Source: CAD feature listing. Evaluate the final solid. Frame: model axes, mm. A direction names the side the tool comes from. Give positions to 0.01 mm unless a question says otherwise; leave off trailing zeros. Loops run counter-clockwise (first coordinate to the right, second up) from the corner with the lowest first, then second, coordinate; pieces in that order, holes last. Notation, with made-up numbers: M 45.5,87.25 L 57.5,87.25 A34 ccw 57.5,122.25 Z; hole C -37,-36 d3. An arc over 180 degrees is marked long. Put each result on its own line as item: value.
from build123d import *

# Parameters (mm, degrees)
F0_R     = 12.5
F1_DEPTH = 20
F2_DEPTH = 5
F3_R     = 7.5
F4_DEPTH = 50


with BuildPart() as f1:
    # F0 (on Front) → F1 (new body, symmetric)
    with BuildSketch(Plane.XZ):
        with BuildLine():
            Line((63.232286, 3.888947), (37.476556, 3.888947))
            ThreePointArc((37.476556, 3.888947), (29.260214, 26.727902), (11.256595, 43.006594))
            ThreePointArc((11.256595, 43.006594), (-55.988459, 23.157086), (-37.272816, -44.412323))
            Line((-37.272816, -44.412323), (-37.272816, -76.111053))
            Line((-37.272816, -76.111053), (-15.272816, -76.111053))
            Line((-15.272816, -76.111053), (-15.272816, -32.970117))
            ThreePointArc((-15.272816, -32.970117), (-12.272816, 30.888947), (-9.272816, -32.970117))
            Line((-9.272816, -32.970117), (-9.272816, -33.111053))
            Line((-9.272816, -33.111053), (-9.272816, -76.111053))
            Line((-9.272816, -76.111053), (12.727184, -76.111053))
            Line((12.727184, -76.111053), (12.727184, -44.412323))
            ThreePointArc((12.727184, -44.412323), (29.722588, -28.247486), (37.476556, -6.111053))
            Line((37.476556, -6.111053), (63.232286, -6.111053))
            ThreePointArc((63.232286, -6.111053), (107.0921, -16.922441), (87.727184, 23.888947))
            ThreePointArc((87.727184, 23.888947), (71.915795, 18.253864), (63.232286, 3.888947))
        make_face()
        with Locations((87.727184, -1.111053)):
            Circle(F0_R, mode=Mode.SUBTRACT)
    extrude(amount=F1_DEPTH, both=True)

    # F0 (on Front) → F2 (join, symmetric)
    with BuildSketch(Plane.XZ):
        with BuildLine():
            ThreePointArc((11.256595, 43.006594), (29.260214, 26.727902), (37.476556, 3.888947))
            Line((37.476556, 3.888947), (63.232286, 3.888947))
            ThreePointArc((63.232286, 3.888947), (71.915795, 18.253864), (87.727184, 23.888947))
            Line((87.727184, 23.888947), (11.256595, 43.006594))
        make_face()
    extrude(amount=F2_DEPTH, both=True)

    # F3 (on Right) → F4 (cut, symmetric)
    with BuildSketch(Plane.YZ):
        with Locations((0, -58.611053)):
            Circle(F3_R)
    extrude(amount=F4_DEPTH, both=True, mode=Mode.SUBTRACT)


solid = f1.part
1. Section query C-C (x = 80). Output: boundary loops of the cut face in (y, z), plus the area to 3 significant figures.
Found:
outline: M -20,-24.89 L 20,-24.89 L 20,-10.94 L -20,-10.94 Z; M -20,8.71 L 20,8.71 L 20,22.66 L 5,22.66 L 5,25.82 L -5,25.82 L -5,22.66 L -20,22.66 Z
area: 1,150 mm^2
2. Access query for faces 5 (the flat face through (-15.273, 0, -50)), 6 (the flat face through (-37.273, 0, -67)), 7 (the flat face through (49, 5, 24)), 8 (the flat face through (12.727, 0, -68)), 9 (the flat face through (49, -5, 24)). Directions: +Z, -Z, +X, -X, +Y, -Y. A direction counts if a zero-diameter tool reaches every point of the face in a straight line with its end or side. Return the directions, or none.
Found:
face 5: -Z, +Y, -Y
face 6: -Z, -X, +Y, -Y
face 7: +Z, +Y
face 8: -Z, +X, +Y, -Y
face 9: +Z, -Y
3. Draft query along Y for faces 1 (the flat face through (51, 12, 3.889)), 2 (the cylindrical face through (1.881, 3.461, -65.265)), 3 (the flat face through (12, -20, -23)), 4 (the flat face through (12, 20, -23)). Return one class per face: pulls with the +Y half, pulls with the -Y half, needs draft (parallel to the pull), parting line crosses it, or undercut.
Found:
face 1: needs draft
face 2: undercut
face 3: pulls with the -Y half
face 4: pulls with the +Y half
4. Material intervals for line 1 (X direction, y = 12.5, z = 0.5); line 2 (X direction, y = -8, z = -66); line 3 (Z direction, x = 4, y = 0), sorted ascending. Write a range as from..to.
Found:
line 1: -62.25..-44.23, 19.69..75.33, 100.12..112.68
line 2: -37.27..-15.27, -9.27..12.73
line 3: -76.11..-66.11, -51.11..-28.66, 26.44..46.17
5. Section query D-D (z = -36.5). Output: boundary loops of the cut face in (x, y).
Found:
outline: M -47.59,-20 L -15.27,-20 L -15.27,20 L -47.59,20 Z; M -9.27,-20 L 23.05,-20 L 23.05,20 L -9.27,20 Z
6. Section query B-B (y = 0). Output: boundary loops of the cut face in (x, z), plus the area to 3 significant figures.
Found:
outline: M -37.27,-76.11 L -15.27,-76.11 L -15.27,-66.11 L -37.27,-66.11 Z; M -37.27,-51.11 L -15.27,-51.11 L -15.27,-32.97 A32 cw long -9.27,-32.97 L -9.27,-51.11 L 12.73,-51.11 L 12.73,-44.41 A50 ccw 37.48,-6.11 L 63.23,-6.11 A25 ccw long 87.73,23.89 L 11.26,43.01 A50 ccw -37.27,-44.41 Z; M -9.27,-76.11 L 12.73,-76.11 L 12.73,-66.11 L -9.27,-66.11 Z; hole C 87.73,-1.11 d25
area: 8,000 mm^2
7. Section query A-A (x = -18). Output: boundary loops of the cut face in (y, z), plus the area to 3 significant figures.
Found:
outline: M -20,-76.11 L 20,-76.11 L 20,-32.59 L -20,-32.59 Z; M -20,30.37 L 20,30.37 L 20,48.56 L -20,48.56 Z; hole C 0,-58.61 d15
area: 2,290 mm^2
8. Contact query for flat-ended pins moving along their axis: P1, Ø6, axis at y = 12, z = -60.5, coming from the +X side; P2, Ø2, axis at y = -14.5, z = -2.5, coming from the -X side; P3, Ø19.5, axis at x = 51.5, z = 22, coming from the -Y side. Output: stop coordinate, or through.
Found:
P1: x = 12.73
P2: x = -62.27
P3: y = -5
